Part model, mm, in its own coordinate system. A direction names the side the tool comes from. Coordinates: 2 decimals unless noted, no trailing zeros. Use a Markdown table: item, result. Add a question column.
1) Drop flat-ended pins along their axis: P1, Ø5, axis at x = 417.5, y = 437, coming from the -Z side; P2, Ø1, axis at y = 426.5, z = 1, coming from the -X side; P3, Ø2, axis at y = 440.5, z = -2.5, coming from the -X side; P4, Ø8, axis at y = 437, z = -1, coming from the -X side. Give the stop position or say it passes through.
2) Probe probe 1 along Y at (x, z) = (416.75, -1.5); probe 2 along Z at (x, y) = (418.5, 433.5); probe 3 along Y at (x, z) = (415.25, -1.5). List the from-to ranges inside material, lowest first. Write a range as [from, to].
3) Tool access for faces 1 (the face through (418.9, 433.63, 0.04)), 2 (the face through (422.53, 425.76, -0.62)), 3 (the face through (412.371, 444.976, -0.827)): list every direction of +Z, -Z, +X, -X, +Y, -Y with a clear straight run to the whole face (end or side of a thin tool).
4) Band-saw the part on A-A (x = 409.75). Give the number of separate pieces and of enclosed holes in the cut face, plus the area to 3 significant figures.
5) Pull direction Y, two halves, no side cores. Call faces 4 (the face through (424, 424.97, 0.04)), 5 (the face through (414.439, 440.906, -0.044)), 6 (the face through (409.82, 429.44, 0.04)): +Y half, -Y half, draft (parallel to the pull), parting line (faces both ways), or undercut.
from build123d import *

# Parameters (mm, degrees)
PLACA_DEPTH                    = 2.5
BUJE_CABLE_PROFILE_R           = 3.5
TORNILLO_PISACABLES_PROFILE_R  = 2.5
PASO_CABLE_PRINCIPAL_PROFILE_R = 1
PESTANA_PROFILE_R              = 1.8
LABIO_PROFILE_R                = 3


with BuildPart() as part:
    # Sk_Placa → Placa (new, symmetric)
    with BuildSketch(Plane(origin=(504.880130221, 233.021598564, 0), x_dir=(0, 0, 1), z_dir=(-0.9079593845004517, -0.41905817746174717, 0))):
        with BuildLine():
            add(Edge.make_bspline(
                [(0, 225.213202705), (1.404685151, 225.213202705), (5.902868455, 222.284529944), (9.072068195, 215.843391455), (6.4788047, 208.217156085), (0, 206.670955869), (-6.4788047, 208.217156085), (-9.072068195, 215.843391455), (-5.902868455, 222.284529944), (-1.404685151, 225.213202705), (0, 225.213202705)],
                knots=[0, 0, 0, 0, 0.085901139, 0.275078775, 0.378517444, 0.5, 0.621482556, 0.724921225, 0.914098861, 1, 1, 1, 1], degree=3))
        make_face()
    extrude(amount=PLACA_DEPTH, both=True)

    # Buje_cable: sweep along a curve in space
    with BuildLine() as buje_cable_path:
        Line((411.620184428, 444.63002849, 0), (415.391708025, 436.458394029, 0))
    # Buje_cable profile (on start of the path) → Buje_cable (sweep)
    with BuildSketch(Plane(origin=(411.620184428, 444.63002849, 0), x_dir=(-0.9079593845004499, -0.4190581774617505, 0), z_dir=(0.41905817746175056, -0.9079593845004501, 0))):
        Circle(BUJE_CABLE_PROFILE_R)
    sweep(path=buje_cable_path.line)

    # Tornillo_pisacables: sweep along a curve in space
    with BuildLine() as tornillo_pisacables_path:
        Line((409.804265659, 429.474091072, 0), (418.883859504, 433.664672846, 0))
    # Tornillo_pisacables profile (on start of the path) → Tornillo_pisacables (sweep)
    with BuildSketch(Plane(origin=(409.804265659, 429.474091072, 0), x_dir=(-0.4190581774617444, 0.9079593845004529, 0), z_dir=(0.9079593845004529, 0.4190581774617444, 0))):
        Circle(TORNILLO_PISACABLES_PROFILE_R)
    sweep(path=tornillo_pisacables_path.line)

    # Paso_cable_principal: sweep along a curve in space
    with BuildLine() as paso_cable_principal_path:
        Line((410.782068073, 446.445947259, 0), (418.325115268, 430.102678338, 0))
    # Paso_cable_principal profile (on start of the path) → Paso_cable_principal (sweep, cut)
    with BuildSketch(Plane(origin=(410.782068073, 446.445947259, 0), x_dir=(-0.9079593845004518, -0.41905817746174673, 0), z_dir=(0.41905817746174673, -0.9079593845004518, 0))):
        Circle(PASO_CABLE_PRINCIPAL_PROFILE_R)
    sweep(path=paso_cable_principal_path.line, mode=Mode.SUBTRACT)

    # Pestana: sweep along a curve in space
    with BuildLine() as pestana_path:
        Line((420.057222401, 422.531693932, 0), (423.325876185, 424.04030337, 0))
    # Pestana profile (on start of the path) → Pestana (sweep)
    with BuildSketch(Plane(origin=(420.057222401, 422.531693932, 0), x_dir=(-0.4190581774617379, 0.9079593845004559, 0), z_dir=(0.9079593845004559, 0.4190581774617379, 0))):
        Circle(PESTANA_PROFILE_R)
    sweep(path=pestana_path.line)

    # Labio: sweep along a curve in space
    with BuildLine() as labio_path:
        Line((423.074441279, 424.585079001, 0), (423.982400663, 425.004137179, 0))
    # Labio profile (on start of the path) → Labio (sweep)
    with BuildSketch(Plane(origin=(423.074441279, 424.585079001, 0), x_dir=(-0.4190581774617578, 0.9079593845004467, 0), z_dir=(0.9079593845004467, 0.4190581774617578, 0))):
        Circle(LABIO_PROFILE_R)
    sweep(path=labio_path.line)


solid = part.part
Answer block:
| question | item | result |
|---|---|---|
| 1 | P1 | z = -3.5 |
| 1 | P2 | x = 412.6 |
| 1 | P3 | x = 409.88 |
| 1 | P4 | x = 408.23 |
| 2 | probe 1 | [420.66, 429.94], [430.48, 434.88], [437.09, 441.06] |
| 2 | probe 2 | [-2.5, 2.5] |
| 2 | probe 3 | [421.25, 434.19], [436.39, 444.31] |
| 3 | face 1 | +Z, -Z, +X |
| 3 | face 2 | none |
| 3 | face 3 | +Z, -Z, -X, +Y |
| 4 | separate pieces | 3 |
| 4 | enclosed holes | 0 |
| 4 | area | 52.3 mm2 |
| 5 | face 4 | +Y half |
| 5 | face 5 | undercut |
| 5 | face 6 | -Y half |
